For this review, take the finished solid that the model builds, in its own axes (mm). Face numbers are marked on the shaded views. A direction names the side the tool comes from. Give positions to 0.01 mm unless a question says otherwise; leave off trailing zeros. Loops run counter-clockwise (first coordinate to the right, second up) from the corner with the lowest first, then second, coordinate; pieces in that order, holes last. Notation, with made-up numbers: (50.5, 28) -> (84.5, 28) arc R20 cw to (84.5, 53) -> close; hole circle Ø7 at (82.5, 6.5). An arc over 180 degrees is marked (long way). Write each question's results on one line, items separated by ' | '. Start each with the question number.
```python
from build123d import *

# Parameters (mm, degrees)
SKETCH1_R           = 1.143
BOSS_EXTRUDE1_DEPTH = 6.35
SKETCH2_R           = 3.81
CUT_EXTRUDE1_DEPTH  = 4.318
SKETCH3_R           = 2.286
CUT_EXTRUDE2_DEPTH  = 4.318
FILLET1_R           = 5.08


with BuildPart() as part:
    # Sketch1 → Boss-Extrude1 (new body)
    with BuildSketch(Plane(origin=(0, 0, 0), x_dir=(1, 0, 0), z_dir=(0, 1, 0))):
        with BuildLine():
            Line((-22.86, 16.51), (22.86, 16.51))
            ThreePointArc((22.86, 16.51), (25.554076836, 15.394076836), (26.67, 12.7))
            Line((26.67, 12.7), (26.67, -12.7))
            ThreePointArc((26.67, -12.7), (25.554076836, -15.394076836), (22.86, -16.51))
            Line((22.86, -16.51), (18.7325, -16.51))
            Line((18.7325, -16.51), (18.7325, -50.165))
            Line((18.7325, -50.165), (-18.7325, -50.165))
            Line((-18.7325, -50.165), (-18.7325, -16.51))
            Line((-18.7325, -16.51), (-22.86, -16.51))
            ThreePointArc((-22.86, -16.51), (-25.554076836, -15.394076836), (-26.67, -12.7))
            Line((-26.67, -12.7), (-26.67, 12.7))
            ThreePointArc((-26.67, 12.7), (-25.554076836, 15.394076836), (-22.86, 16.51))
        make_face()
        with Locations((-23.241, 13.208)):
            Circle(SKETCH1_R, mode=Mode.SUBTRACT)
        with Locations((23.241, 13.208)):
            Circle(SKETCH1_R, mode=Mode.SUBTRACT)
        with Locations((23.241, -13.208)):
            Circle(SKETCH1_R, mode=Mode.SUBTRACT)
        with Locations((-23.50753981, -13.208)):
            Circle(SKETCH1_R, mode=Mode.SUBTRACT)
        with Locations((14.224, -34.925)):
            Circle(SKETCH1_R, mode=Mode.SUBTRACT)
        with Locations((-14.224, -34.925)):
            Circle(SKETCH1_R, mode=Mode.SUBTRACT)
    extrude(amount=BOSS_EXTRUDE1_DEPTH)

    # Sketch2 → Cut-Extrude1 (cut)
    with BuildSketch(Plane.XZ):
        Circle(SKETCH2_R)
    extrude(amount=-CUT_EXTRUDE1_DEPTH, mode=Mode.SUBTRACT)

    # Sketch3 → Cut-Extrude2 (cut)
    with BuildSketch(Plane(origin=(0, 4.318, 0), x_dir=(-1, 0, 0), z_dir=(0, -1, 0))):
        Circle(SKETCH3_R)
    extrude(amount=-CUT_EXTRUDE2_DEPTH, mode=Mode.SUBTRACT)

    # Fillet1
    fillet1_edges = [part.edges().sort_by_distance(p)[0] for p in [
        (-18.7325, 3.175, 16.51),
        (18.7325, 3.175, 16.51),
        (18.7325, 3.175, 50.165),
        (-18.7325, 3.175, 50.165),
    ]]
    fillet(fillet1_edges, radius=FILLET1_R)


solid = part.part
```
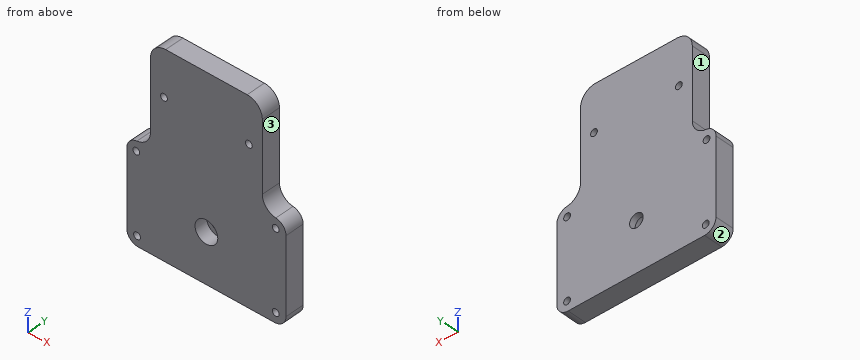
1. Wall thickness on L1, parallel to Z at x = 0, y = 5.65 (3 decimals); L2, parallel to X at y = 1.5, z = 35; L3, parallel to X at y = 3.75, z = 34.5: over which ranges is each line inside the solid? List them lowest first.
2. We need section D-D (y = 2). Count the separate pieces of the cut face and the enclosed holes in it, plus the area to 3 significant figures.
3. We need section A-A (z = 0). Write out the cut boundary in (x, y).
4. We need section B-B (x = 0). Write out the cut boundary in (y, z) (3 decimals).
5. We need section C-C (z = 39). Write out the cut boundary in (x, y).
6. For pin 1 Ø3 at (y, z) = (2.5, 34.5) entering from +X; pin 2 Ø1.8 at (x, z) = (23.241, 13.208) entering from +Y; pin 3 Ø2.5 at (x, z) = (0.5, 2) entering from -Y, all flat-tipped, find the tip position at first contact; note any pin that passes through.
7. Machinability: for the marked faces 1, 2 and 3, which of the approach directions +Z, -Z, +X, -X, +Y, -Y give a long, thin tool a straight path to every point of the face, cutting with its end or side? Answer none if there is none.
Response:
1) L1: z = -16.51 to -2.286, 2.286 to 50.165 | L2: x = -18.73 to -15.36, -13.08 to 13.08, 15.36 to 18.73 | L3: x = -18.73 to -15.29, -13.16 to 13.16, 15.29 to 18.73
2) separate pieces: 1 | enclosed holes: 7 | area: 2,940 mm2
3) outline: (-26.67, 0) -> (-3.81, 0) -> (-3.81, 4.32) -> (-2.29, 4.32) -> (-2.29, 6.35) -> (-26.67, 6.35) -> close; (2.29, 4.32) -> (3.81, 4.32) -> (3.81, 0) -> (26.67, 0) -> (26.67, 6.35) -> (2.29, 6.35) -> close
4) outline: (0, -16.51) -> (6.35, -16.51) -> (6.35, -2.286) -> (4.318, -2.286) -> (4.318, -3.81) -> (0, -3.81) -> close; (0, 3.81) -> (4.318, 3.81) -> (4.318, 2.286) -> (6.35, 2.286) -> (6.35, 50.165) -> (0, 50.165) -> close
5) outline: (-18.73, 0) -> (18.73, 0) -> (18.73, 6.35) -> (-18.73, 6.35) -> close
6) pin 1: stops at x = 18.73 | pin 2: passes through | pin 3: stops at y = 4.32
7) face 1: +Z, -X, +Y, -Y | face 2: -Z, -X, +Y, -Y | face 3: +Z, +X, +Y, -Y
